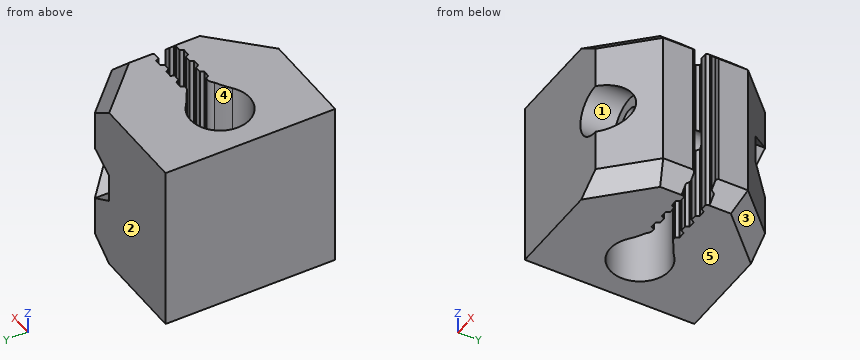
```python
from build123d import *

# Parameters (mm, degrees)
BOSS_EXTRUDE1_DEPTH = 19.8
FILLET1_R           = 10
FILLET2_R           = 1
CHAMFER1_SIZE       = 5
CUT_EXTRUDE1_REACH  = 35.956
SKETCH2_R           = 1.6
SKETCH3_R           = 3
CUT_EXTRUDE2_DEPTH  = 4
CUT_EXTRUDE3_DEPTH  = 4
CHAMFER2_SIZE       = 2


with BuildPart() as part:
    # Sketch1 → Boss-Extrude1 (new body)
    with BuildSketch(Plane.XY):
        with BuildLine():
            Line((18.861664867, 11.25), (18.111664867, 11.25))
            Line((18.111664867, 11.25), (17.886664867, 11.65))
            Line((17.886664867, 11.65), (17.086664867, 11.65))
            Line((17.086664867, 11.65), (16.861664867, 11.25))
            Line((16.861664867, 11.25), (16.111664867, 11.25))
            Line((16.111664867, 11.25), (15.886664867, 11.65))
            Line((15.886664867, 11.65), (15.086664867, 11.65))
            Line((15.086664867, 11.65), (14.861664867, 11.25))
            Line((14.861664867, 11.25), (14.111664867, 11.25))
            Line((14.111664867, 11.25), (13.886664867, 11.65))
            Line((13.886664867, 11.65), (13.086664867, 11.65))
            Line((13.086664867, 11.65), (12.861664867, 11.25))
            Line((12.861664867, 11.25), (12.111664867, 11.25))
            Line((12.111664867, 11.25), (11.886664867, 11.65))
            Line((11.886664867, 11.65), (11.086664867, 11.65))
            Line((11.086664867, 11.65), (10.861664867, 11.25))
            Line((10.861664867, 11.25), (10.111664867, 11.25))
            Line((10.111664867, 11.25), (9.886664867, 11.65))
            Line((9.886664867, 11.65), (9.086664867, 11.65))
            ThreePointArc((9.086664867, 11.65), (2.5, 10), (9.086664867, 8.35))
            Line((9.086664867, 8.35), (9.886664867, 8.35))
            Line((9.886664867, 8.35), (10.111664867, 8.75))
            Line((10.111664867, 8.75), (10.861664867, 8.75))
            Line((10.861664867, 8.75), (11.086664867, 8.35))
            Line((11.086664867, 8.35), (11.886664867, 8.35))
            Line((11.886664867, 8.35), (12.111664867, 8.75))
            Line((12.111664867, 8.75), (12.861664867, 8.75))
            Line((12.861664867, 8.75), (13.086664867, 8.35))
            Line((13.086664867, 8.35), (13.886664867, 8.35))
            Line((13.886664867, 8.35), (14.111664867, 8.75))
            Line((14.111664867, 8.75), (14.861664867, 8.75))
            Line((14.861664867, 8.75), (15.086664867, 8.35))
            Line((15.086664867, 8.35), (15.886664867, 8.35))
            Line((15.886664867, 8.35), (16.111664867, 8.75))
            Line((16.111664867, 8.75), (16.861664867, 8.75))
            Line((16.861664867, 8.75), (17.086664867, 8.35))
            Line((17.086664867, 8.35), (17.886664867, 8.35))
            Line((17.886664867, 8.35), (18.111664867, 8.75))
            Line((18.111664867, 8.75), (18.861664867, 8.75))
            Line((18.861664867, 8.75), (19, 8.504070874))
            Line((19, 8.504070874), (19, 0))
            Line((19, 0), (0, 0))
            Line((0, 0), (0, 20))
            Line((0, 20), (19, 20))
            Line((19, 20), (19, 11.495929126))
            Line((19, 11.495929126), (18.861664867, 11.25))
        make_face()
    extrude(amount=BOSS_EXTRUDE1_DEPTH)

    # Fillet1
    # the kernel refuses this fillet: 10 mm, written as the material it takes off along each edge
    with BuildSketch(Plane(origin=(9.086664867, 8.35, -3.562523753), x_dir=(1, 0, 0), z_dir=(0, 0, 1))) as fillet1_piece_1:
        with BuildLine():
            CenterArc((5.295321975, -8.932641286), FILLET1_R, 116.713674189, 11.667329514)
            Line((-0.913557167, -1.093647741), (-1.03773475, -0.93686787))
            ThreePointArc((-1.03773475, -0.93686787), (-0.554023827, -0.465591965), (-0.17638085, 0.094285714))
            Line((-0.17638085, 0.094285714), (0, 0.2))
            ThreePointArc((0, 0.2), (0.4, 0.2), (0.710093561, 0.178652826))
            Line((0.710093561, 0.178652826), (0.8, 0))
        make_face()
    extrude(amount=26.925047506, mode=Mode.SUBTRACT)
    with BuildSketch(Plane(origin=(9.086664867, 11.65, -3.562523753), x_dir=(1, 0, 0), z_dir=(0, 0, 1))) as fillet1_piece_2:
        with BuildLine():
            CenterArc((5.295321975, 8.932641286), FILLET1_R, 231.618996297, 11.667329514)
            Line((-0.913557167, 1.093647741), (-1.03773475, 0.93686787))
            ThreePointArc((-1.03773475, 0.93686787), (-0.554023827, 0.465591965), (-0.17638085, -0.094285714))
            Line((-0.17638085, -0.094285714), (0, -0.2))
            ThreePointArc((0, -0.2), (0.4, -0.2), (0.710093561, -0.178652826))
            Line((0.710093561, -0.178652826), (0.8, 0))
        make_face()
    extrude(amount=26.925047506, mode=Mode.SUBTRACT)

    # Fillet2
    # the kernel refuses this fillet: 1 mm, written as the material it takes off along each edge
    with BuildSketch(Plane(origin=(10.111664867, 8.75, -1.4375), x_dir=(-0.4902612396325597, -0.8715755371245488, 0), z_dir=(0, 0, 1))) as fillet2_piece_1:
        with BuildLine():
            CenterArc((0.589675324, 0.991417173), FILLET2_R, 209.357753543, 53.130102354)
            Line((-0.281900213, 0.501155934), (-0.299331724, 0.491350709))
            Line((-0.299331724, 0.491350709), (-0.017431511, -0.009805225))
            Line((-0.017431511, -0.009805225), (0, -0.02))
            ThreePointArc((0, -0.02), (0.229469497, -0.02), (0.456324267, -0.019828343))
            Line((0.456324267, -0.019828343), (0.458938994, 0))
        make_face()
    extrude(amount=22.675, mode=Mode.SUBTRACT)
    with BuildSketch(Plane(origin=(10.111664867, 11.25, -1.4375), x_dir=(-0.4902612396325682, 0.8715755371245442, 0), z_dir=(0, 0, 1))) as fillet2_piece_2:
        with BuildLine():
            CenterArc((0.589675324, -0.991417173), FILLET2_R, 97.512144103, 53.130102354)
            Line((-0.281900213, -0.501155934), (-0.299331724, -0.491350709))
            Line((-0.299331724, -0.491350709), (-0.017431511, 0.009805225))
            Line((-0.017431511, 0.009805225), (0, 0.02))
            ThreePointArc((0, 0.02), (0.229469497, 0.02), (0.456324267, 0.019828343))
            Line((0.456324267, 0.019828343), (0.458938994, 0))
        make_face()
    extrude(amount=22.675, mode=Mode.SUBTRACT)

    # Chamfer1
    chamfer1_edges = [part.edges().sort_by_distance(p)[0] for p in [
        (19, 20, 9.9),
        (19, 0, 9.9),
    ]]
    chamfer(chamfer1_edges, length=CHAMFER1_SIZE)

    # Cut-Extrude1: up to this face of the body (flat: up to its plane)
    cut_extrude1_end = Plane(part.part.faces().sort_by_distance((7, 20, 9.9))[0])
    # Sketch2 → Cut-Extrude1 (cut, up to the picked face)
    with BuildSketch(Plane.XZ, mode=Mode.PRIVATE) as cut_extrude1_sk1:
        with Locations(Location((14, 9.9, 0), (0, 0, 270))):
            Circle(SKETCH2_R)
    cut_extrude1_tool1 = split(extrude(cut_extrude1_sk1.sketch, amount=-CUT_EXTRUDE1_REACH, mode=Mode.PRIVATE), bisect_by=cut_extrude1_end, keep=Keep.BOTH, mode=Mode.PRIVATE)
    add(cut_extrude1_tool1.solids().sort_by(Axis((14, 0, 9.9), (0, 1, 0)))[0], mode=Mode.SUBTRACT)

    # Sketch3 → Cut-Extrude2 (cut)
    with BuildSketch(Plane.XZ):
        with Locations(Location((14, 9.9, 0), (0, 0, 270))):
            Circle(SKETCH3_R)
    extrude(amount=-CUT_EXTRUDE2_DEPTH, mode=Mode.SUBTRACT)

    # Sketch4 → Cut-Extrude3 (cut)
    with BuildSketch(Plane(origin=(0, 20, 0), x_dir=(1, 0, 0), z_dir=(0, 1, 0))):
        Polygon((11.15, -8.254551733), (11.15, -11.545448267), (14, -13.190896534), (16.85, -11.545448267), (16.85, -8.254551733), (14, -6.609103466), align=None)
    extrude(amount=-CUT_EXTRUDE3_DEPTH, mode=Mode.SUBTRACT)

    # Chamfer2
    chamfer2_edges = [part.edges().sort_by_distance(p)[0] for p in [
        (16.5, 2.5, 0),
        (19, 6.752035437, 0),
        (16.5, 17.5, 0),
        (19, 13.247964563, 0),
        (16.5, 17.5, 19.8),
        (19, 13.247964563, 19.8),
        (19, 6.752035437, 19.8),
        (16.5, 2.5, 19.8),
    ]]
    chamfer(chamfer2_edges, length=CHAMFER2_SIZE)


solid = part.part
```
Source: CAD feature listing. Evaluate the final solid. Frame: model axes, mm. Face numbers are marked on the shaded views. A direction names the side the tool comes from. Coordinates: 2 decimals unless noted, no trailing zeros. Write each loop counter-clockwise with the first axis right and the second up, starting at its lowest first coordinate (ties: lowest second). Pieces come first, ordered by that corner, then holes. Notation, with made-up numbers: (29, 81.5) - (86, 81.5) arc R30 cw to (86, 115.5) - close; hole circle Ø10 at (20, 32). An arc over 180 degrees is marked (long way). Answer as a JSON object with one key per item and string values.
Q1. Section query B-B, the plane z = 9.9. State how many separate pieces and enclosed holes the cut face has, plus the area to 3 significant figures.
Ans:
{"separate pieces": "3", "enclosed holes": "0", "area": "221 mm2"}
Q2. Section query C-C, the plane y = 4.5. Output: boundary loops of the cut face in (x, z).
Ans:
{"outline": "(0, 0) - (15.67, 0) - (18.5, 2) - (18.5, 17.8) - (15.67, 19.8) - (0, 19.8) - close; hole circle Ø3.2 at (14, 9.9)"}
Q3. Set-up query: the marked faces 4 and 5. Return all of +Z, -Z, +X, -X, +Y, -Y with unobstructed straight access to the full face (end or side cutting, diameter ignored); none if empty.
Ans:
{"face 4": "+Z, -Z", "face 5": "-Z, +X, -X, +Y, -Y"}
Q4. Material intervals for line 1 (Y direction, x = 15.5, z = 11); line 2 (Z direction, x = 14, y = 6.9); line 3 (X direction, y = 13, z = 9.5), sorted ascending. Write a range as [from, to].
Ans:
{"line 1": "y = [4, 8.35], [11.65, 16]", "line 2": "z = [0, 8.3], [11.5, 19.8]", "line 3": "x = [0, 4.2], [7.8, 12.45], [15.55, 19]"}
Q5. First-contact query: pin 1 Ø1.9 at (x, z) = (14, 9.9) entering from -Y; pin 2 Ø1 at (y, z) = (18.5, 9.5) entering from +X; pin 3 Ø0.8 at (x, z) = (14.5, 16.5) entering from -Y; pin 4 Ø0.6 at (x, z) = (18.5, 7.5) entering from -Y. Flat tips, straight axial feed; report the tip coordinate or a pass-through.
Ans:
{"pin 1": "passes through", "pin 2": "stops at x = 11.15", "pin 3": "stops at y = 0.1", "pin 4": "stops at y = 4.2"}
Q6. Draft query along X for the marked faces 1, 2 and 3. Return one class per face: released by +X, released by -X, zero draft, split by the parting line, or undercut.
Ans:
{"face 1": "undercut", "face 2": "zero draft", "face 3": "released by +X"}
Q7. Section query A-A, the plane x = 6. Output: boundary loops of the cut face in (y, z), plus the area to 3 significant figures.
Ans:
{"outline": "(0, 0) - (6.5, 0) - (6.5, 19.8) - (0, 19.8) - close; (13.5, 0) - (20, 0) - (20, 19.8) - (13.5, 19.8) - close", "area": "257 mm2"}
Q8. Section query D-D, the plane y = 1.5. Output: boundary loops of the cut face in (x, z).
Ans:
{"outline": "(0, 0) - (12.67, 0) - (15.5, 2) - (15.5, 7.3) arc R3 cw (long way) to (15.5, 12.5) - (15.5, 17.8) - (12.67, 19.8) - (0, 19.8) - close"}
